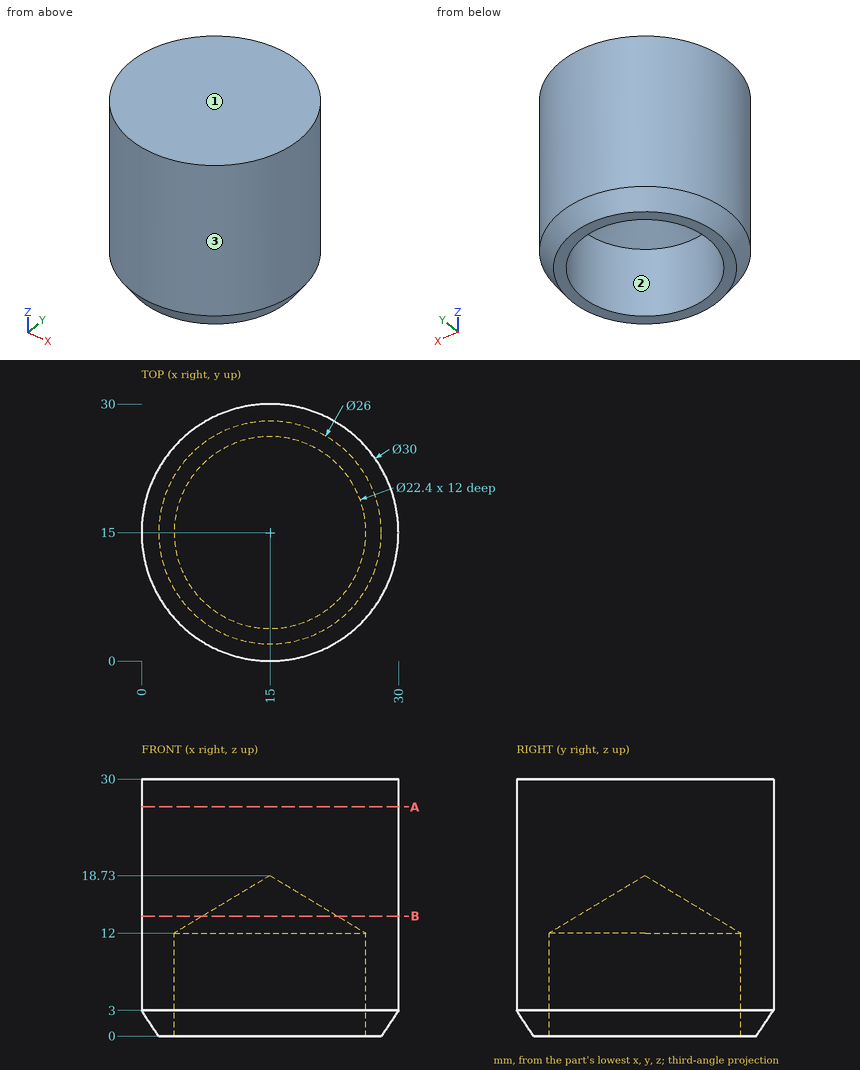
Part print with two shaded views. Sizes in mm from the minimum x, y, z corner. Round coordinates to 2 decimals unless told otherwise and drop trailing zeros. Order: outer loops, then holes, each group sorted by start corner. A loop starts at its lowest first (then second) coordinate and runs counter-clockwise, first axis right, second up. Notation, with made-up numbers: M 82.25,11 L 92.25,11 A25 ccw 92.25,45 Z; hole C -38,42.5 d2. An arc over 180 degrees is marked long. Answer in a Markdown table with one row per item. Add a question column.
Q1. Pin check, flat tips, straight feed: pin 1 (1 mm diameter, centred on y = 10.5, z = 11, fed in from -X); pin 2 (1 mm diameter, centred on y = 9.5, z = 7.5, fed in from -X); pin 3 (1 mm diameter, centred on y = 19.5, z = 6.5, fed in from +X). Stop position of each tip, or through.
Q2. Wall check: L1, parallel to Y at x = 15, z = 4.25; L2, parallel to X at y = 15.5, z = 28.25; L3, parallel to X at y = 19, z = 28.25. Give the ranges that are in metal, low to high. Write a range as from..to.
Q3. Mould opens along X. For the marked faces 1, 2 and 3 say: +X half, -X half, draft (parallel to the pull), parting line (faces both ways), or undercut.
Q4. Cut at B-B on z = 14. Give the cut face in (x, y).
Q5. Cut at A-A on z = 26.75. Give the cut face in (x, y).
Established:
| question | item | result |
|---|---|---|
| 1 | pin 1 | stops at x = 0.54 |
| 1 | pin 2 | stops at x = 0.86 |
| 1 | pin 3 | stops at x = 29.46 |
| 2 | L1 | y = 0..3.8, 26.2..30 |
| 2 | L2 | x = 0.01..29.99 |
| 2 | L3 | x = 0.54..29.46 |
| 3 | face 1 | draft |
| 3 | face 2 | undercut |
| 3 | face 3 | parting line |
| 4 | outline | C 15,15 d30; hole C 15,15 d15.74 |
| 5 | outline | C 15,15 d30 |
